Source: CAD feature listing. Evaluate the final solid. Frame: model axes, mm. A direction names the side the tool comes from. Give positions to 0.01 mm unless a question says otherwise; leave off trailing zeros. Write each loop counter-clockwise with the first axis right and the second up, starting at its lowest first coordinate (ties: lowest second). Pieces come first, ordered by that corner, then holes. Notation, with made-up numbers: (-1.75, 10.5) -> (6.25, 10.5) arc R17 cw to (6.25, 21.5) -> close; hole circle Ø2 at (-10, 18.25). An arc over 180 degrees is marked (long way). Write item = value, one per line.
from build123d import *

# Parameters (mm, degrees)
SKETCH_1_W      = 70
SKETCH_1_H      = 70
SKETCH_1_W_2    = 64
SKETCH_1_H_2    = 64
EXTRUDE_1_DEPTH = 150
FILLET_1_R      = 2


with BuildPart() as part:
    # 草图1 → 凸台-拉伸1 (new body)
    with BuildSketch(Plane.XY):
        Rectangle(SKETCH_1_W, SKETCH_1_H)
        Rectangle(SKETCH_1_W_2, SKETCH_1_H_2, mode=Mode.SUBTRACT)
    extrude(amount=EXTRUDE_1_DEPTH)

    # 圆角1
    fillet_1_edges = [part.edges().sort_by_distance(p)[0] for p in [
        (32, -32, 75),
        (32, 32, 75),
        (-32, 32, 75),
        (-32, -32, 75),
        (35, -35, 75),
        (-35, -35, 75),
        (-35, 35, 75),
        (35, 35, 75),
    ]]
    fillet(fillet_1_edges, radius=FILLET_1_R)


solid = part.part
(1) Access query for faces 5 (the face through (0, -32, 74)), 6 (the face through (-35, 0, 74)). Directions: +Z, -Z, +X, -X, +Y, -Y. A direction counts if a zero-diameter tool reaches every point of the face in a straight line with its end or side. Return the directions, or none.
Values follow:
face_5 = +Z, -Z
face_6 = +Z, -Z, -X, +Y, -Y
(2) Material intervals for line 1 (Y direction, x = 12, z = 85.5); line 2 (X direction, y = 30.5, z = 28.5), sorted ascending.
Values follow:
line_1 = -35 to -32, 32 to 35
line_2 = -35 to -31.94, 31.94 to 35
(3) Pull-direction query (Y, two-part tool) for faces 1 (the face through (0, 35, 74)), 2 (the face through (-32, 0, 74)), 3 (the face through (0, -35, 74)), 4 (the face through (32, 0, 74)); classes: pulls with the +Y half, pulls with the -Y half, needs draft (parallel to the pull), parting line crosses it, or undercut.
Values follow:
face_1 = pulls with the +Y half
face_2 = undercut
face_3 = pulls with the -Y half
face_4 = undercut
(4) Section query C-C (z = 76). Return loops of the section in (x, y), plus the area to 3 significant figures.
Values follow:
outline = (-35, -33) arc R2 ccw to (-33, -35) -> (33, -35) arc R2 ccw to (35, -33) -> (35, 33) arc R2 ccw to (33, 35) -> (-33, 35) arc R2 ccw to (-35, 33) -> close; hole (-32, -30) arc R2 ccw to (-30, -32) -> (30, -32) arc R2 ccw to (32, -30) -> (32, 30) arc R2 ccw to (30, 32) -> (-30, 32) arc R2 ccw to (-32, 30) -> close
area = 804 mm2
(5) Section query A-A (y = -22). Return loops of the section in (x, z), plus the area to 3 significant figures.
Values follow:
outline = (-35, 0) -> (-32, 0) -> (-32, 150) -> (-35, 150) -> close; (32, 0) -> (35, 0) -> (35, 150) -> (32, 150) -> close
area = 900 mm2
